Could you check a few things on this model? Use its own coordinates, in mm. Face numbers are marked on the shaded views. Coordinates: 2 decimals unless noted, no trailing zeros. Order: outer loops, then holes, each group sorted by start corner. A loop starts at its lowest first (then second) coordinate and runs counter-clockwise, first axis right, second up. Notation, with made-up numbers: (-15, 71.5) -> (-7, 71.5) arc R24 cw to (-7, 82.5) -> close; hole circle Ø10 at (41.25, 48.5). An arc over 180 degrees is marked (long way). Use a Markdown table: item, result. Add a question column.
1) If we section it at B-B (y = 0): Write out the boundary of the cut face in (x, z), plus the area to 3 significant figures.
2) If we section it at A-A (z = 20): Write out the boundary of the cut face in (x, y).
3) If we section it at D-D (z = 10): Write out the boundary of the cut face in (x, y).
4) If we section it at C-C (x = 0): Write out the boundary of the cut face in (y, z), plus the area to 3 significant figures.
5) Thinking about a two-plate mould opening in Y: for the marked faces 1, 2 and 3, which applies, +Y half, -Y half, draft (parallel to the pull), parting line (faces both ways), or undercut?
6) If I drill on L1, parallel to X at y = 0, z = 31; L2, parallel to X at y = 31, z = 38; L3, parallel to Y at x = -5.25, z = 31.5, over which ranges is the centre line in solid material (lowest first)? Write a range as [from, to].
7) Will these pins go through, and if not, where does the flat tip stop? pin 1 Ø2 at (x, y) = (1, 75) entering from -Z; pin 2 Ø6 at (y, z) = (19.62, 10.3) entering from +X; pin 3 Ø8.5 at (y, z) = (19.62, 29.7) entering from -X; pin 4 Ø5 at (x, z) = (-8, 16) entering from -Y.
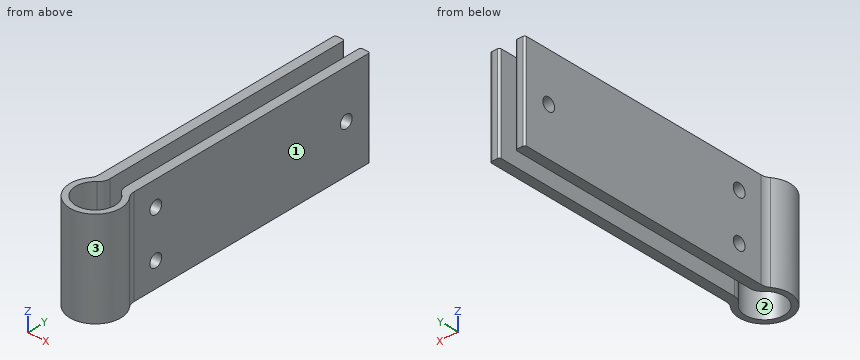
```python
from build123d import *

# Parameters (mm, degrees)
BOSS_EXTRU_1_DEPTH = 40
CONG_1_R           = 5
CONG_2_R           = 0.8
D_GAGEMENT_M1_61_D = 5.4


with BuildPart() as part:
    # Esquisse1 → Boss.-Extru.1 (new body)
    with BuildSketch(Plane.XY):
        with BuildLine():
            Line((-3.266012474, 7.466971442), (-3.266012474, 117.466971442))
            Line((-3.266012474, 117.466971442), (-7.266012474, 117.466971442))
            Line((-7.266012474, 117.466971442), (-7.266012474, 7.649023646))
            ThreePointArc((-7.266012474, 7.649023646), (0, -10.55), (7.266012474, 7.649023646))
            Line((7.266012474, 7.649023646), (7.266012474, 117.466971442))
            Line((7.266012474, 117.466971442), (3.266012474, 117.466971442))
            Line((3.266012474, 117.466971442), (3.266012474, 7.466971442))
            ThreePointArc((3.266012474, 7.466971442), (0, -8.15), (-3.266012474, 7.466971442))
        make_face()
    extrude(amount=BOSS_EXTRU_1_DEPTH)

    # Congé1
    cong_1_edges = [part.edges().sort_by_distance(p)[0] for p in [
        (7.266012474, 7.649023646, 20),
        (-7.266012474, 7.649023646, 20),
        (-3.266012474, 7.466971442, 20),
        (3.266012474, 7.466971442, 20),
    ]]
    fillet(cong_1_edges, radius=CONG_1_R)

    # Congé2
    cong_2_edges = [part.edges().sort_by_distance(p)[0] for p in [
        (3.266012474, 117.466971442, 20),
        (7.266012474, 117.466971442, 20),
        (-7.266012474, 117.466971442, 20),
        (-3.266012474, 117.466971442, 20),
    ]]
    fillet(cong_2_edges, radius=CONG_2_R)

    # Dégagement M1.61 (through all)
    with Locations(Plane.ZY.offset(7.266012474)):
        with Locations((20, 106.594477776), (10.299577014, 19.622753657), (29.700422986, 19.622753657)):
            Hole(D_GAGEMENT_M1_61_D / 2)


solid = part.part
```
Answer sheet:
| question | item | result |
|---|---|---|
| 1 | outline | (-10.55, 0) -> (-8.15, 0) -> (-8.15, 40) -> (-10.55, 40) -> close; (8.15, 0) -> (10.55, 0) -> (10.55, 40) -> (8.15, 40) -> close |
| 1 | area | 192 mm2 |
| 2 | outline | (-8.32, 6.48) arc R10.55 ccw (long way) to (8.32, 6.48) arc R5 cw to (7.27, 9.56) -> (7.27, 103.89) -> (3.27, 103.89) -> (3.27, 10.23) arc R5 ccw to (5.12, 6.34) arc R8.15 cw (long way) to (-5.12, 6.34) arc R5 ccw to (-3.27, 10.23) -> (-3.27, 103.89) -> (-7.27, 103.89) -> (-7.27, 9.56) arc R5 cw to start; (-7.27, 109.29) -> (-3.27, 109.29) -> (-3.27, 116.67) arc R0.8 ccw to (-4.07, 117.47) -> (-6.47, 117.47) arc R0.8 ccw to (-7.27, 116.67) -> close; (3.27, 109.29) -> (7.27, 109.29) -> (7.27, 116.67) arc R0.8 ccw to (6.47, 117.47) -> (4.07, 117.47) arc R0.8 ccw to (3.27, 116.67) -> close |
| 3 | outline | (-8.32, 6.48) arc R10.55 ccw (long way) to (8.32, 6.48) arc R5 cw to (7.27, 9.56) -> (7.27, 16.94) -> (3.27, 16.94) -> (3.27, 10.23) arc R5 ccw to (5.12, 6.34) arc R8.15 cw (long way) to (-5.12, 6.34) arc R5 ccw to (-3.27, 10.23) -> (-3.27, 16.94) -> (-7.27, 16.94) -> (-7.27, 9.56) arc R5 cw to start; (-7.27, 22.31) -> (-3.27, 22.31) -> (-3.27, 116.67) arc R0.8 ccw to (-4.07, 117.47) -> (-6.47, 117.47) arc R0.8 ccw to (-7.27, 116.67) -> close; (3.27, 22.31) -> (7.27, 22.31) -> (7.27, 116.67) arc R0.8 ccw to (6.47, 117.47) -> (4.07, 117.47) arc R0.8 ccw to (3.27, 116.67) -> close |
| 4 | outline | (-10.55, 0) -> (-8.15, 0) -> (-8.15, 40) -> (-10.55, 40) -> close |
| 4 | area | 96.0 mm2 |
| 5 | face 1 | draft |
| 5 | face 2 | undercut |
| 5 | face 3 | parting line |
| 6 | L1 | [-10.55, -8.15], [8.15, 10.55] |
| 6 | L2 | [-7.27, -3.27], [3.27, 7.27] |
| 6 | L3 | [-9.15, -6.23], [6.23, 17.61], [21.64, 117.47] |
| 7 | pin 1 | through |
| 7 | pin 2 | x = 7.27 |
| 7 | pin 3 | x = -7.27 |
| 7 | pin 4 | y = -9 |
